Input: part model. Units: mm. Frame: model coordinates. A direction names the side the tool comes from. Give positions to 0.01 mm unless a question says otherwise; leave off trailing zeros. Loops run counter-clockwise (first coordinate to the right, second up) from the corner with the lowest first, then second, coordinate; pieces in that order, holes last. Notation, with made-up numbers: M -10.5,83.25 L 36.5,83.25 A19 ccw 36.5,95.25 Z; hole C 75,57 d9. An arc over 180 degrees is marked long. Return JSON: item names as keys, results as strings. Group by question number.
```python
from build123d import *

# Parameters (mm, degrees)
F0_R     = 8.5
F1_DEPTH = 2
F3_D     = 6
F4_W     = 5
F4_H     = 2
F5_DEPTH = 2.001


with BuildPart() as f1:
    # F0 (on Top) → F1 (new body)
    with BuildSketch(Plane.XY):
        Circle(F0_R)
    extrude(amount=-F1_DEPTH)

    # F3 (through all)
    with Locations(Plane.XY):
        with Locations((4.242641, -4.242641), (-4.242641, 4.242641)):
            Hole(F3_D / 2)

    # F4 (on face) → F5 (cut, through all)
    with BuildSketch(Plane.XY):
        with Locations((-3.5, -1)):
            Rectangle(F4_W, F4_H)
        with Locations((3.5, 1)):
            Rectangle(F4_W, F4_H)
    extrude(amount=-F5_DEPTH, mode=Mode.SUBTRACT)


solid = f1.part
```
Item 1: Section A-A, the plane x = 2. Return loops of the section in (y, z).
Item 2: Reachability of faces 4 (the face through (0, 0, -2)), 5 (the face through (-6, -1, -1)) from +Z, -Z, +X, -X, +Y, -Y: full face, straight path, thin tool, end or side. Return the list, or none.
Item 3: Pull-direction query (Y, two-part tool) for faces 1 (the face through (0, 0, 0)), 2 (the face through (-4, -2, -1)), 3 (the face through (-6.12, -5.9, -0.99)); classes: pulls with the +Y half, pulls with the -Y half, needs draft (parallel to the pull), parting line crosses it, or undercut.
Item 4: Material intervals for line 1 (X direction, y = 0.25, z = -0.5); line 2 (Y direction, x = -1.75, z = -0.35); line 3 (X direction, y = 1.5, z = -0.95), sorted ascending. Write a range as from..to.
Item 5: Section C-C, the plane x = 5. Return loops of the section in (y, z).
Item 6: First-contact query: pin 1 Ø1 at (x, z) = (3.5, -0.5) entering from +Y; pin 2 Ø0.6 at (x, z) = (2.5, -1.5) entering from -Y; pin 3 Ø0.6 at (x, z) = (-3, -0.5) entering from +Y. Flat tips, straight axial feed; report the tip coordinate or a pass-through.
Item 7: Section B-B, the plane y = -2.25. Return loops of the section in (x, z).
Item 8: Section D-D, the plane z = -1.05. Return loops of the section in (x, y), then the cut area to 3 significant figures.
Answer below:
{
 "1": {"outline": "M -8.26,-2 L -6.24,-2 L -6.24,0 L -8.26,0 Z; M -2.25,-2 L 0,-2 L 0,0 L -2.25,0 Z; M 2,-2 L 8.26,-2 L 8.26,0 L 2,0 Z"},
 "2": {"face 4": "-Z, +X, -X, +Y, -Y", "face 5": "+Z, -Z"},
 "3": {"face 1": "needs draft", "face 2": "undercut", "face 3": "parting line crosses it"},
 "4": {"line 1": "-8.5..1, 6..8.5", "line 2": "-8.32..-2, 0..2.57, 5.91..8.32", "line 3": "-8.37..-5.46, -3.03..1, 6..8.37"},
 "5": {"outline": "M -1.34,-2 L 0,-2 L 0,0 L -1.34,0 Z; M 2,-2 L 6.87,-2 L 6.87,0 L 2,0 Z"},
 "6": {"pin 1": "y = 7.95", "pin 2": "y = -8.21", "pin 3": "y = 8.06"},
 "7": {"outline": "M -8.2,-2 L 2,-2 L 2,0 L -8.2,0 Z; M 6.49,-2 L 8.2,-2 L 8.2,0 L 6.49,0 Z"},
 "8": {"outline": "M -7.23,4.46 A8.5 ccw 4.46,-7.23 A3 cw long 7.23,-4.46 A8.5 ccw -4.46,7.23 A3 cw long Z; hole M -6,-2 L -1,-2 L -1,0 L -6,0 Z; hole M 1,0 L 6,0 L 6,2 L 1,2 Z", "area": "153 mm^2"}
}
